```python
from build123d import *

# Parameters (mm, degrees)
SKETCH2_R           = 10
SKETCH2_R_2         = 2.5
BOSS_EXTRUDE1_DEPTH = 40
BOSS_EXTRUDE2_START = 40
SKETCH2_3_R         = 2.5
BOSS_EXTRUDE2_DEPTH = 50
SKETCH3_R           = 5
CUT_EXTRUDE1_DEPTH  = 20


with BuildPart() as part:
    # Sketch2 → Boss-Extrude1 (new body)
    # profile 1 of 2: a face of its own
    with BuildSketch(Plane(origin=(0, 0, 0), x_dir=(1, 0, 0), z_dir=(0, 1, 0))):
        with Locations(Location((0, 0, 0), (0, 0, 270))):
            Circle(SKETCH2_R)
        Circle(SKETCH2_R_2, mode=Mode.SUBTRACT)
    # profile 2 of 2: a face of its own
    with BuildSketch(Plane(origin=(0, 0, 0), x_dir=(1, 0, 0), z_dir=(0, 1, 0))):
        Circle(SKETCH2_R_2)
    extrude(amount=BOSS_EXTRUDE1_DEPTH)

    # Sketch2<3> → Boss-Extrude2 (add)
    with BuildSketch(Plane(origin=(0, 0, 0), x_dir=(1, 0, 0), z_dir=(0, 1, 0)).offset(BOSS_EXTRUDE2_START)):
        with Locations(Location((0, 0, 0), (0, 0, 270))):
            Circle(SKETCH2_3_R)
    extrude(amount=BOSS_EXTRUDE2_DEPTH)

    # Sketch3 → Cut-Extrude1 (cut)
    with BuildSketch(Plane(origin=(0, 0, 0), x_dir=(1, 0, 0), z_dir=(0, 1, 0))):
        with Locations(Location((0, 0, 0), (0, 0, 270))):
            Circle(SKETCH3_R)
    extrude(amount=CUT_EXTRUDE1_DEPTH, mode=Mode.SUBTRACT)


solid = part.part
```
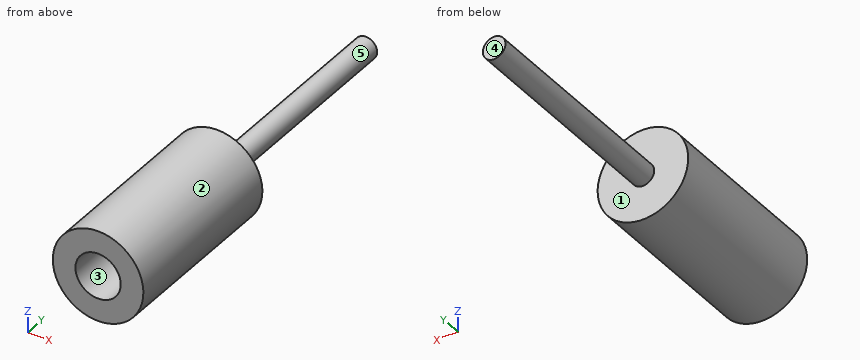
Here's how the part is built. I have some questions about the finished solid (model axes, mm). Face numbers are marked on the shaded views. A direction names the side the tool comes from. Coordinates: 2 decimals unless noted, no trailing zeros. Write each loop counter-clockwise with the first axis right and the second up, starting at its lowest first coordinate (ties: lowest second). Pieces come first, ordered by that corner, then holes. Notation, with made-up numbers: (-1, 55) -> (30, 55) arc R29 cw to (30, 88) -> close; hole circle Ø9 at (-1.5, 85.5). An arc over 180 degrees is marked (long way). Use a Markdown table: item, result. Add a question column.
(1) Please list where these lines run through material, in increasing order: line 1 (X direction, y = 13.5, z = 0); line 2 (Y direction, x = 1.5, z = 1.5); line 3 (Y direction, x = -4.5, z = -1).
(2) If we section it at B-B, the plane x = 0: Write out the boundary of the cut face in (y, z).
(3) We'd pull the mould along Z, two halves only. Please class the marked faces 1, 2 and 3: +Z half, -Z half, draft (parallel to the pull), parting line (faces both ways), or undercut.
(4) If we section it at D-D, the plane y = 47: Write out the boundary of the cut face in (x, z), and give its area (3 significant figures).
(5) For the marked faces 4 and 5, which set-ups out of +Z, -Z, +X, -X, +Y, -Y let a thin tool reach every point of the face, with its end or its side?
(6) I'm going to push flat-ended pins straight in: P1, Ø1, axis at x = 5.5, y = 12.5, coming from the +Z side; P2, Ø1.5, axis at y = 44, z = 0, coming from the +X side; P3, Ø8, axis at x = -8, y = 13.5, coming from the -Z side. Where does each tip first touch, or does it pass through?
(7) If we section it at C-C, the plane y = 15: Write out the boundary of the cut face in (x, z), and give its area (3 significant figures).
(8) If we section it at A-A, the plane z = 0: Write out the boundary of the cut face in (x, y).
Outcome:
| question | item | result |
|---|---|---|
| 1 | line 1 | x = -10 to -5, 5 to 10 |
| 1 | line 2 | y = 20 to 90 |
| 1 | line 3 | y = 20 to 40 |
| 2 | outline | (0, -10) -> (40, -10) -> (40, -2.5) -> (90, -2.5) -> (90, 2.5) -> (40, 2.5) -> (40, 10) -> (0, 10) -> (0, 5) -> (20, 5) -> (20, -5) -> (0, -5) -> close |
| 3 | face 1 | draft |
| 3 | face 2 | parting line |
| 3 | face 3 | undercut |
| 4 | outline | circle Ø5 at (0, 0) |
| 4 | area | 19.6 mm^2 |
| 5 | face 4 | +Z, -Z, +X, -X, +Y |
| 5 | face 5 | +Y |
| 6 | P1 | stops at z = 8.66 |
| 6 | P2 | stops at x = 2.5 |
| 6 | P3 | stops at z = -9.17 |
| 7 | outline | circle Ø20 at (0, 0); hole circle Ø10 at (0, 0) |
| 7 | area | 236 mm^2 |
| 8 | outline | (-10, 0) -> (-5, 0) -> (-5, 20) -> (5, 20) -> (5, 0) -> (10, 0) -> (10, 40) -> (2.5, 40) -> (2.5, 90) -> (-2.5, 90) -> (-2.5, 40) -> (-10, 40) -> close |
